Here's the drawing with two shaded views (mm, measured from the low corner). I have some questions. A direction names the side the tool comes from. Round coordinates to 2 decimals unless told otherwise and drop trailing zeros. Order: outer loops, then holes, each group sorted by start corner. A loop starts at its lowest first (then second) coordinate and runs counter-clockwise, first axis right, second up.
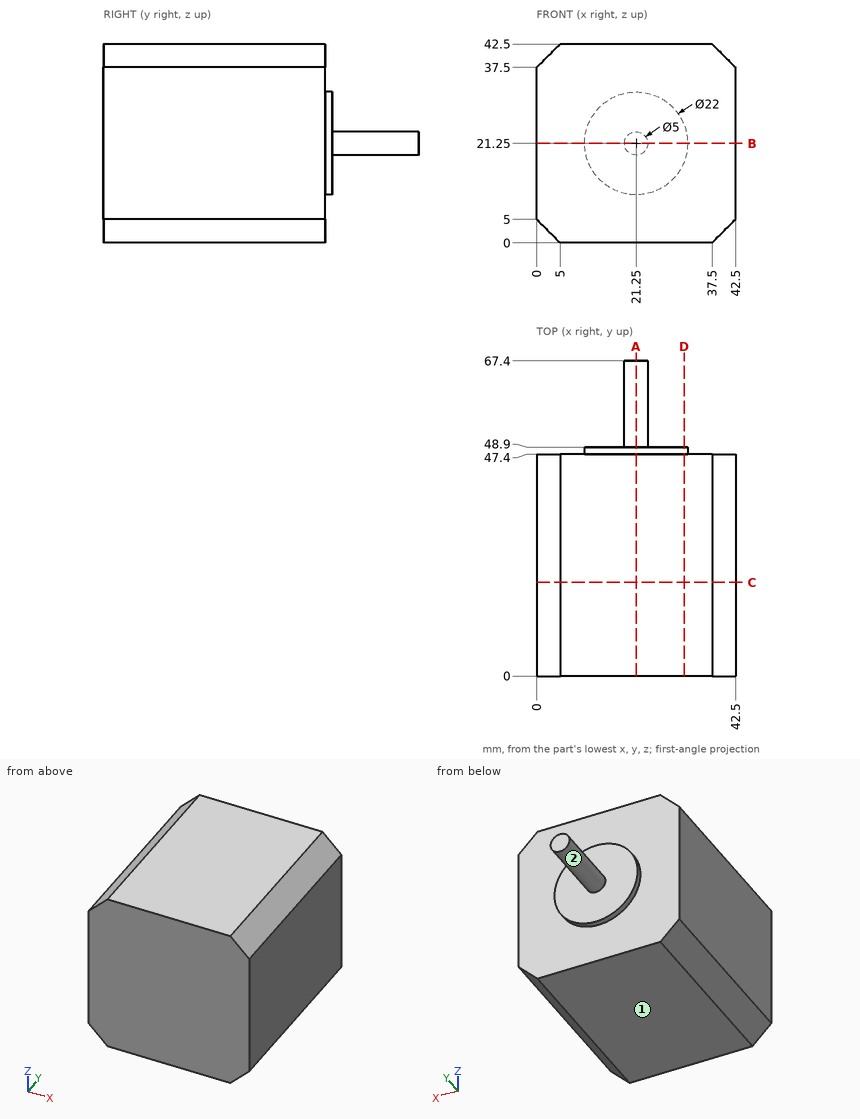
1. If we section it at C-C, the plane y = 20: Write out the boundary of the cut face in (x, z).
Evaluation:
outline: (0, 5) - (5, 0) - (37.5, 0) - (42.5, 5) - (42.5, 37.5) - (37.5, 42.5) - (5, 42.5) - (0, 37.5) - close
2. If we section it at B-B, the plane z = 21.25: Write out the boundary of the cut face in (x, y), and give its area (3 significant figures).
Evaluation:
outline: (0, 0) - (42.5, 0) - (42.5, 47.4) - (32.25, 47.4) - (32.25, 48.9) - (23.75, 48.9) - (23.75, 67.4) - (18.75, 67.4) - (18.75, 48.9) - (10.25, 48.9) - (10.25, 47.4) - (0, 47.4) - close
area: 2,140 mm2
3. On a 3-axis mill with a long thin cutter (end or side, diameter ignored), from which of +Z, -Z, +X, -X, +Y, -Y can I reach the whole of each face in a straight line? I mean the marked faces 1 and 2. Say none if no direction works.
Evaluation:
face 1: -Z, +X, -X, +Y, -Y
face 2: +Y
4. If we section it at D-D, the plane x = 31.5: Write out the boundary of the cut face in (y, z).
Evaluation:
outline: (0, 0) - (47.4, 0) - (47.4, 17.26) - (48.9, 17.26) - (48.9, 25.24) - (47.4, 25.24) - (47.4, 42.5) - (0, 42.5) - close
5. I'm going to push a flat-ended pin straight in: P1, Ø10, axis at x = 31, z = 30, coming from the +Y side. Where does the tip first touch, or does it pass through?
Evaluation:
P1: stops at y = 48.9
6. If we section it at A-A, the plane x = 21.25: Write out the boundary of the cut face in (y, z).
Evaluation:
outline: (0, 0) - (47.4, 0) - (47.4, 10.25) - (48.9, 10.25) - (48.9, 18.75) - (67.4, 18.75) - (67.4, 23.75) - (48.9, 23.75) - (48.9, 32.25) - (47.4, 32.25) - (47.4, 42.5) - (0, 42.5) - close
7. I need wall thicknesses on probe 1 along Y at (x, z) = (36, 13.5); probe 2 along Y at (x, z) = (16.5, 12); probe 3 along Z at (x, y) = (40, 4.5). Which ranges of each line are inside material? Lowest first, please.
Evaluation:
probe 1: y = 0 to 47.4
probe 2: y = 0 to 48.9
probe 3: z = 2.5 to 40
